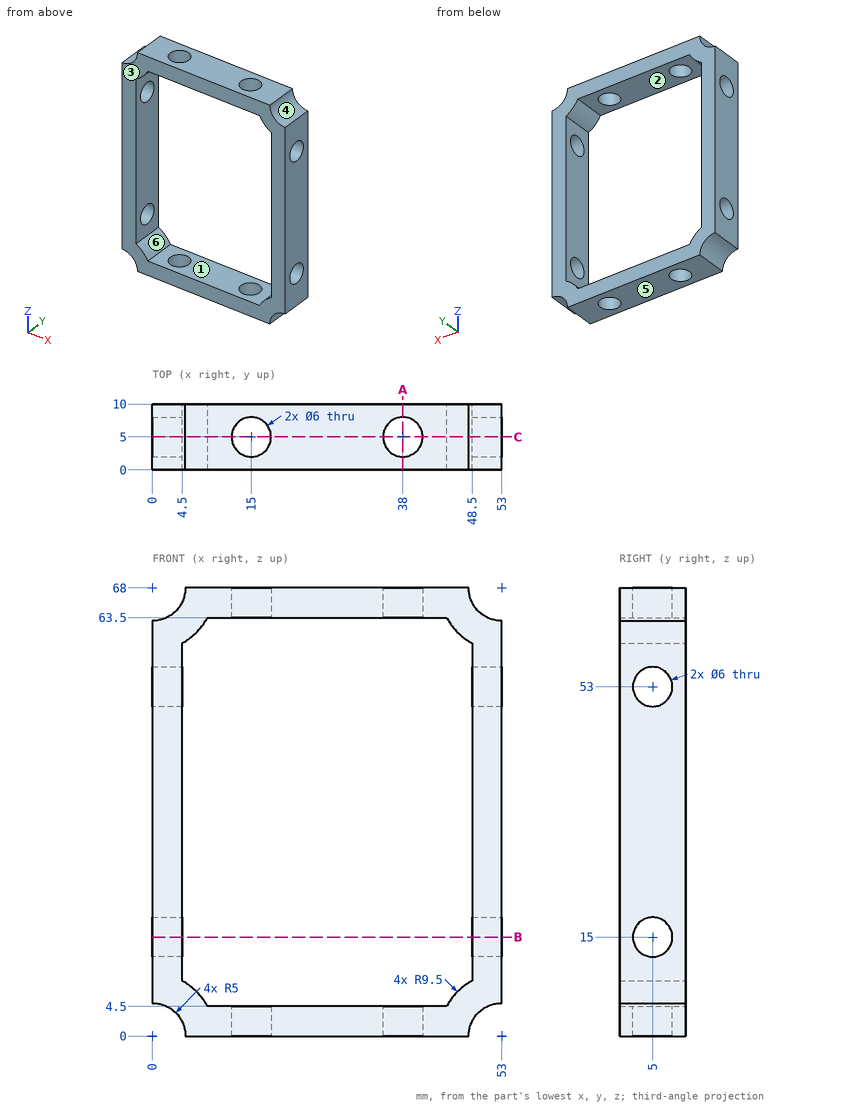
Study the drawing (mm; zero at the part's minimum x, y, z) and answer. A direction names the side the tool comes from. Give positions to 0.01 mm unless a question says otherwise; leave off trailing zeros. Order: outer loops, then holes, each group sorted by start corner. A loop starts at its lowest first (then second) coordinate and runs counter-clockwise, first axis right, second up. Notation, with made-up numbers: (35.25, 36) - (88.25, 36) arc R17 cw to (88.25, 66) - close; hole circle Ø9 at (-32.75, 71). An arc over 180 degrees is marked (long way). Answer in a Markdown table with one row per item. Add a question column.
Q1. The part is cut by section A-A (x = 38). Determine the outline of the cut face in (y, z).
Q2. Find the intervals of material crossed by line 1 along X through (y, z) = (2.25, 48); line 2 along Y through (x, z) = (15, 2.8); line 3 along Z through (x, y) = (50, 3.75), in increasing order. Write a range as [from, to].
Q3. The part is cut by section C-C (y = 5). Give the number of separate pieces and of enclosed holes in the cut face, then the cut area to 3 significant figures.
Q4. For a pull along Z with two mould halves and no side action, classify the marked faces 1, 2, 3 and 4 as released by +Z, released by -Z, zero draft, split by the parting line, or undercut.
Q5. The part is cut by section B-B (z = 15). Determine the outline of the cut face in (x, y).
Q6. Which of the six approach directions +Z, -Z, +X, -X, +Y, -Y give full straight-line access (tool end or side, diameter ignored) to the marked faces 5 and 6?
Determined:
| question | item | result |
|---|---|---|
| 1 | outline | (0, 0) - (2, 0) - (2, 4.5) - (0, 4.5) - close; (0, 63.5) - (2, 63.5) - (2, 68) - (0, 68) - close; (8, 0) - (10, 0) - (10, 4.5) - (8, 4.5) - close; (8, 63.5) - (10, 63.5) - (10, 68) - (8, 68) - close |
| 2 | line 1 | x = [0, 4.5], [48.5, 53] |
| 2 | line 2 | y = [0, 2], [8, 10] |
| 2 | line 3 | z = [4, 12.27], [17.73, 50.27], [55.73, 64] |
| 3 | separate pieces | 8 |
| 3 | enclosed holes | 0 |
| 3 | area | 749 mm² |
| 4 | face 1 | undercut |
| 4 | face 2 | undercut |
| 4 | face 3 | zero draft |
| 4 | face 4 | released by +Z |
| 5 | outline | (0, 0) - (4.5, 0) - (4.5, 2) - (0, 2) - close; (0, 8) - (4.5, 8) - (4.5, 10) - (0, 10) - close; (48.5, 0) - (53, 0) - (53, 2) - (48.5, 2) - close; (48.5, 8) - (53, 8) - (53, 10) - (48.5, 10) - close |
| 6 | face 5 | -Z, +X, -X, +Y, -Y |
| 6 | face 6 | +Y, -Y |
